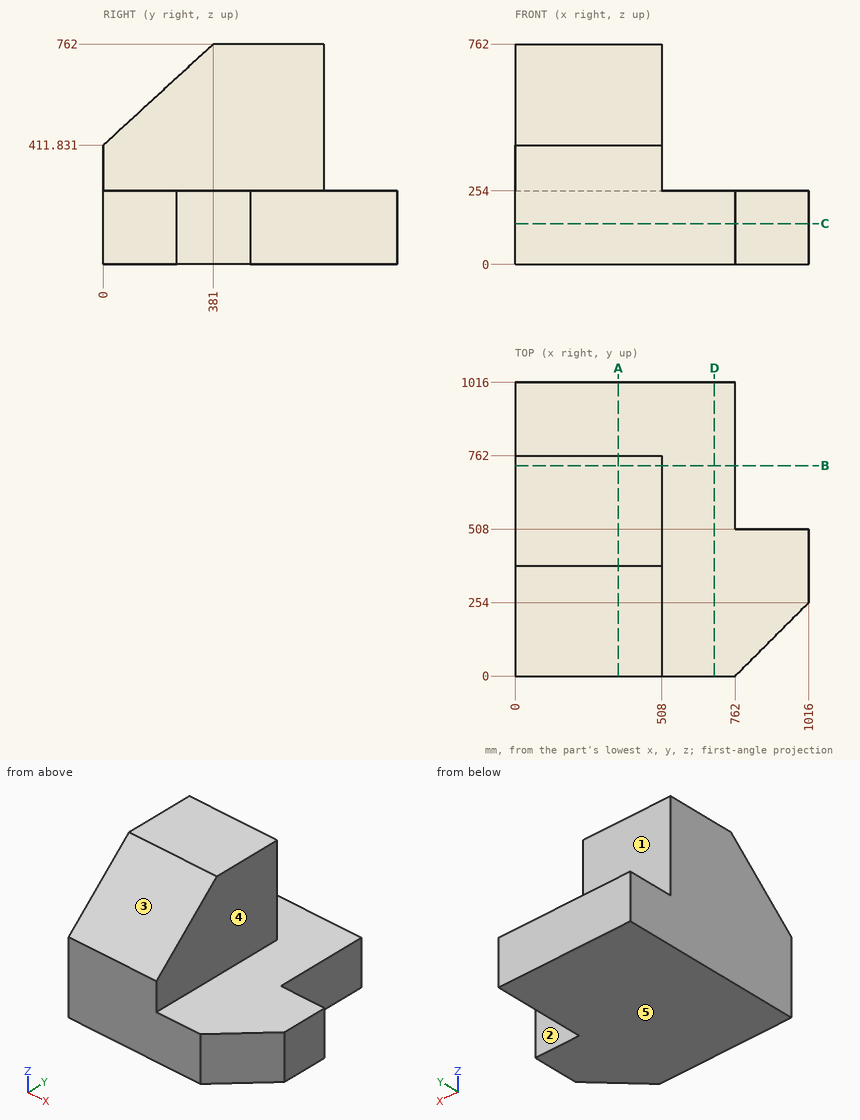
Answer from the drawing. Dimensions are ordinates in mm from the lowest x, y and z of the part. A direction names the side the tool comes from. Round coordinates to 2 decimals unless told otherwise and drop trailing zeros. Order: outer loops, then holes, each group sorted by start corner. A loop starts at its lowest first (then second) coordinate and runs counter-clockwise, first axis right, second up.
1) The part is cut by section A-A on x = 357.5. Write down the section's boundary in (y, z).
2) Flat-ended cylindrical pins translate along their axes: pin 1 (1 mm diameter, centred on x = 607.5, y = 904, fed in from +Z); pin 2 (6 mm diameter, centred on x = 127, z = 364, fed in from +Y). Find the tip coordinate at first contact, or state that the pin passes through.
3) For the marked faces 1, 2, 3, 4 and 5, determine the directions among +Z, -Z, +X, -X, +Y, -Y from which every point of the face is accessible in a straight line to the end or side of a thin tool.
4) The part is cut by section D-D on x = 690. Write down the section's boundary in (y, z), plus the area to 3 significant figures.
5) Straight lines are drawn through the part: L1, parallel to X at y = 400, z = 526.5; L2, parallel to Z at x = 753.5, y = 380; L3, parallel to X at y = 649.5, z = 107. For each, find the intervals that lie inside material, in ascending order.
6) The part is cut by section B-B on y = 727.5. Write down the section's boundary in (x, z).
7) The part is cut by section C-C on z = 141. Write down the section's boundary in (x, y), plus the area to 3 significant figures.
Resolved:
1. outline: (0, 0) - (1016, 0) - (1016, 254) - (762, 254) - (762, 762) - (381, 762) - (0, 411.83) - close
2. pin 1: stops at z = 254
2. pin 2: stops at y = 762
3. face 1: +Z, +X, -X, +Y
3. face 2: +Z, -Z, +X, +Y
3. face 3: +Z, +X, -X, -Y
3. face 4: +Z, +X, +Y, -Y
3. face 5: -Z, +X, -X, +Y, -Y
4. outline: (0, 0) - (1016, 0) - (1016, 254) - (0, 254) - close
4. area: 258,000 mm2
5. L1: x = 0 to 508
5. L2: z = 0 to 254
5. L3: x = 0 to 762
6. outline: (0, 0) - (762, 0) - (762, 254) - (508, 254) - (508, 762) - (0, 762) - close
7. outline: (0, 0) - (762, 0) - (1016, 254) - (1016, 508) - (762, 508) - (762, 1016) - (0, 1016) - close
7. area: 871,000 mm2
